```python
from build123d import *

# Parameters (mm, degrees)
F1_DEPTH = 127
F2_SIZE  = 14.2875
F3_R     = 12.7
F4_DEPTH = 273.05


with BuildPart() as f1:
    # F0 (on Front) → F1 (new body)
    with BuildSketch(Plane.XZ):
        Polygon((0, 101.6), (0, 0), (304.8, 0), (304.8, 101.6), (266.7, 101.6), (266.7, 38.1), (31.75, 38.1), (31.75, 101.6), align=None)
    extrude(amount=F1_DEPTH)

    # F2
    f2_edges = [f1.edges().sort_by_distance(p)[0] for p in [
        (0, -63.5, 101.6),
    ]]
    chamfer(f2_edges, length=F2_SIZE)

    # F3 (on face) → F4 (cut)
    with BuildSketch(Plane.YZ.offset(304.8)):
        with BuildLine():
            ThreePointArc((-85.389287, 90.112113), (-76.216845, 98.544213), (-64.138096, 101.6))
            Line((-64.138096, 101.6), (-127, 101.6))
            Line((-127, 101.6), (-127, 50.8))
            Line((-127, 50.8), (-111.125, 50.8))
            Line((-111.125, 50.8), (-85.389287, 90.112113))
        make_face()
        with BuildLine():
            Line((-15.875, 50.8), (0, 50.8))
            Line((0, 50.8), (0, 101.6))
            Line((0, 101.6), (-64.138096, 101.6))
            ThreePointArc((-64.138096, 101.6), (-51.747613, 98.372865), (-42.505615, 89.51149))
            Line((-42.505615, 89.51149), (-15.875, 50.8))
        make_face()
        with Locations((-64.138096, 76.2)):
            Circle(F3_R)
        Polygon((-76.2, 16.51), (-76.2, 0), (-50.8, 0), (-50.8, 16.51), (-31.75, 16.51), (-31.75, 29.21), (-50.8, 29.21), (-50.8, 38.1), (-76.2, 38.1), (-76.2, 29.21), (-95.25, 29.21), (-95.25, 16.51), align=None)
    extrude(amount=-F4_DEPTH, mode=Mode.SUBTRACT)


solid = f1.part
```
Part model, mm, in its own coordinate system. A direction names the side the tool comes from. Round coordinates to 2 decimals unless told otherwise and drop trailing zeros. Loops run counter-clockwise (first coordinate to the right, second up) from the corner with the lowest first, then second, coordinate; pieces in that order, holes last.
Item 1: Cut at B-B, the plane x = 263.5. Give the cut face in (y, z), then the cut area to 3 significant figures.
Item 2: Drop flat-ended pins along their axis: P1, Ø21, axis at x = 192, y = -84, coming from the +Z side; P2, Ø4, axis at y = -16, z = 70.5, coming from the +X side; P3, Ø7.5, axis at x = 282.5, y = -67, coming from the -Z side. Give the stop position or say it passes through.
Item 3: Mould opens along Z. For faces 1 (the face through (170, -95.25, 23)), 2 (the face through (170, -41, 16.51)), 3 (the face through (304.8, -63, 39)), 4 (the face through (286.02, -98.44, 70.18)) say: +Z half, -Z half, draft (parallel to the pull), parting line (faces both ways), or undercut.
Item 4: Drill centre lines: line 1 (Z direction, x = 199.5, y = -38); line 2 (X direction, y = -36.5, z = 46); line 3 (Y direction, x = 211, z = 20.5). Where is each one in solid material? Low to high.
Item 5: Cut at D-D, the plane y = -115. Give the cut face in (x, z), then the cut area to 3 significant figures.
Item 6: 3-axis set-ups, long thin cutter, end or side, ignore diameter. For faces 5 (the face through (151, -25, 38.1)), 6 (the face through (286, -8, 50.8)), 7 (the face through (23, -63, 101.6)), 8 (the face through (286.02, -58.28, 64.93)): which of +Z, -Z, +X, -X, +Y, -Y reach the whole face in a straight line?
Item 7: Cut at A-A, the plane z = 47.5. Give the cut face in (x, y), then the cut area to 3 significant figures.
Item 8: Cut at C-C, the plane z = 79. Give the cut face in (x, y).
A:
1. outline: (-127, 0) - (-76.2, 0) - (-76.2, 16.51) - (-95.25, 16.51) - (-95.25, 29.21) - (-76.2, 29.21) - (-76.2, 38.1) - (-127, 38.1) - close; (-50.8, 0) - (0, 0) - (0, 38.1) - (-50.8, 38.1) - (-50.8, 29.21) - (-31.75, 29.21) - (-31.75, 16.51) - (-50.8, 16.51) - close
1. area: 3,390 mm2
2. P1: stops at z = 38.1
2. P2: stops at x = 31.75
2. P3: stops at z = 38.1
3. face 1: undercut
3. face 2: undercut
3. face 3: draft
3. face 4: +Z half
4. line 1: z = 0 to 16.51, 29.21 to 38.1
4. line 2: x = 0 to 31.75, 266.7 to 304.8
4. line 3: y = -127 to -95.25, -31.75 to 0
5. outline: (0, 0) - (304.8, 0) - (304.8, 50.8) - (266.7, 50.8) - (266.7, 38.1) - (31.75, 38.1) - (31.75, 101.6) - (14.29, 101.6) - (0, 87.31) - close
5. area: 14,000 mm2
6. face 5: +Z, +Y, -Y
6. face 6: +Z, +X, +Y
6. face 7: +Z, +X, -X, +Y, -Y
6. face 8: +X
7. outline: (0, -127) - (31.75, -127) - (31.75, 0) - (0, 0) - close; (266.7, -127) - (304.8, -127) - (304.8, 0) - (266.7, 0) - close
7. area: 8,870 mm2
8. outline: (0, -127) - (31.75, -127) - (31.75, 0) - (0, 0) - close; (266.7, -92.66) - (304.8, -92.66) - (304.8, -76.53) - (266.7, -76.53) - close; (266.7, -51.75) - (304.8, -51.75) - (304.8, -35.27) - (266.7, -35.27) - close
